Drawing for the job (mm, zero at the part's lowest x, y, z). A direction names the side the tool comes from. Give positions to 0.01 mm unless a question says otherwise; leave off trailing zeros. Order: outer loops, then holes, each group sorted by start corner. A loop starts at its lowest first (then second) coordinate and runs counter-clockwise, first axis right, second up. Notation, with made-up numbers: (45.5, -30.75) - (87.5, -30.75) arc R4 ccw to (87.5, -24.75) - close; hole circle Ø3 at (20.25, 12). An arc over 180 degrees is marked (long way). Write each question's results on one line, items separated by ' | '. Start each with the question number.
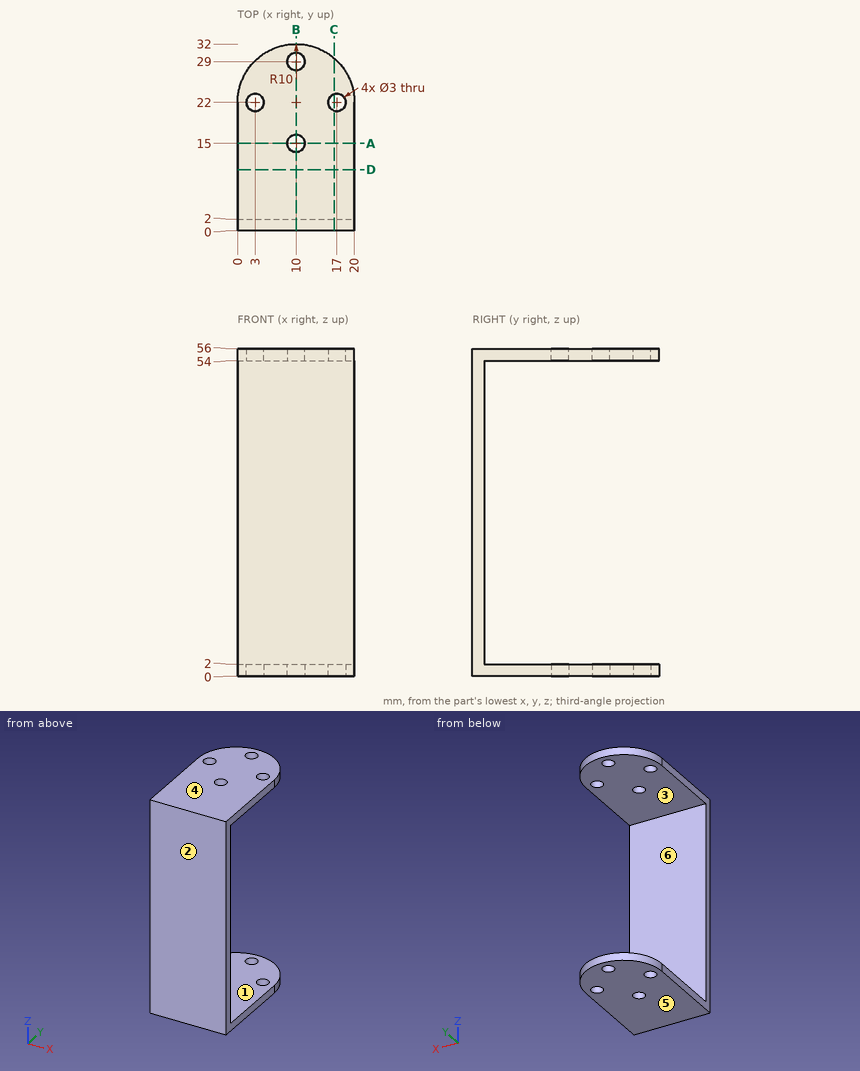
Item 1: Cut at A-A, the plane y = 15. List the corners of the cut face in (x, z), then the cut area to 3 significant figures.
Item 2: Probe line 1 along X through (y, z) = (22, 0.4); line 2 along Y through (x, z) = (10, 55.45); line 3 along Z through (x, y) = (10, 26). List the from-to ranges inside material, lowest first. Write a range as from..to.
Item 3: Cut at D-D, the plane y = 10.5. List the corners of the cut face in (x, z).
Item 4: Two-plate mould, pull along Z, no slides. Class the marked faces 3, 4, 5 and 6: +Z half, -Z half, draft (parallel to the pull), parting line (faces both ways), or undercut.
Item 5: Cut at C-C, the plane x = 16.5. List the corners of the cut face in (y, z), then the cut area to 3 significant figures.
Item 6: Cut at B-B, the plane x = 10. List the corners of the cut face in (y, z).
Item 7: Which spindle directions (+Z, -Z, +X, -X, +Y, -Y) get a long thin tool onto all of the face, cutting with end or side? Do the marked faces 1 and 2. Say none if no direction does.
Item 8: Flat gauge pins, fed straight in: pin 1 Ø1.5 at (x, z) = (5, 30.5) entering from -Y; pin 2 Ø8 at (x, z) = (14.5, 50.5) entering from +Y. Where does each tip first touch, or does it go through?
Values found:
1) outline: (0, 0) - (8.5, 0) - (8.5, 2) - (0, 2) - close; (0, 54) - (8.5, 54) - (8.5, 56) - (0, 56) - close; (11.5, 0) - (20, 0) - (20, 2) - (11.5, 2) - close; (11.5, 54) - (20, 54) - (20, 56) - (11.5, 56) - close | area: 68.0 mm2
2) line 1: x = 0..1.5, 4.5..15.5, 18.5..20 | line 2: y = 0..13.5, 16.5..27.5, 30.5..32 | line 3: z = 0..2, 54..56
3) outline: (0, 0) - (20, 0) - (20, 2) - (0, 2) - close; (0, 54) - (20, 54) - (20, 56) - (0, 56) - close
4) face 3: undercut | face 4: +Z half | face 5: -Z half | face 6: undercut
5) outline: (0, 0) - (20.59, 0) - (20.59, 2) - (2, 2) - (2, 54) - (20.59, 54) - (20.59, 56) - (0, 56) - close; (23.41, 0) - (29.6, 0) - (29.6, 2) - (23.41, 2) - close; (23.41, 54) - (29.6, 54) - (29.6, 56) - (23.41, 56) - close | area: 211 mm2
6) outline: (0, 0) - (13.5, 0) - (13.5, 2) - (2, 2) - (2, 54) - (13.5, 54) - (13.5, 56) - (0, 56) - close; (16.5, 0) - (27.5, 0) - (27.5, 2) - (16.5, 2) - close; (16.5, 54) - (27.5, 54) - (27.5, 56) - (16.5, 56) - close; (30.5, 0) - (32, 0) - (32, 2) - (30.5, 2) - close; (30.5, 54) - (32, 54) - (32, 56) - (30.5, 56) - close
7) face 1: +X, -X, +Y | face 2: +Z, -Z, +X, -X, -Y
8) pin 1: stops at y = 0 | pin 2: stops at y = 31.67
